Autodesk Inventor part; units mm, degrees
ref_plane "YZ Plane" through (0, 0, 0) normal (1, 0, 0) x (0, 1, 0)
ref_plane "XZ Plane" through (0, 0, 0) normal (0, 1, 0) x (-1, 0, 0)
ref_plane "XY Plane" through (0, 0, 0) normal (0, 0, 1) x (1, 0, 0)
sketch "Sketch1" plane through (0, 0, 0) normal (0, 1, 0) x (-1, 0, 0)
  line L0 (0, 0) -> (100, 0)
  line L1 (100, 0) -> (100, -50)
  line L2 (100, -50) -> (0, -50)
  line L3 (0, -50) -> (0, 0)
  line L4 (0, 0) -> (0, -16.6667)
  line L5 (0, -16.6667) -> (6, -16.6667)
  dimension "d0" = 100
  dimension "d1" = 50
  dimension "d2" = 16.6667
  dimension "d3" = 6
extrude "Extrusion1" add sketch "Sketch1" along normal blind 6
sketch "Sketch3" plane through (0, 6, 0) normal (0, 1, 0) x (1, 0, 0)
  circle A0 centre (-13, 12.5) radius 2.75
  line L0 (0, 0) -> (0, 50)
  line L1 (-100, 0) -> (0, 0)
  circle A1 centre (-13, 37.5) radius 2.75
  dimension "d21" = 5.5
  dimension "d22" = 13
  dimension "d23" = 12.5
  dimension "d26" = 25
extrude "Extrusion3" cut sketch "Sketch3" against normal through all
sketch "Sketch4" plane through (0, 6, 0) normal (0, 1, 0) x (1, 0, 0)
  circle A0 centre (-13, 12.5) radius 2.75
  line L0 (-13, 12.5) -> (-73, 12.5)
  line L1 (-73, 12.5) -> (-91, 12.5) construction
  line L2 (-73, 15.25) -> (-91, 15.25)
  line L3 (-91, 9.75) -> (-73, 9.75)
  arc A1 (-73, 9.75) -> (-73, 15.25) centre (-73, 12.5) ccw
  arc A2 (-91, 15.25) -> (-91, 9.75) centre (-91, 12.5) ccw
  point P0 (0, 0)
  point P1 (-82, 12.5)
  dimension "d33" = 60
  dimension "d34" = 18
  dimension "d35" = 5.5
extrude "Extrusion4" cut sketch "Sketch4" against normal through all contours A1 L3 A2 L2
pattern_linear "Rectangular Pattern2" count 2 spacing 25 along (0, 0, -1) of "Extrusion4"
sketch "Sketch5" plane through (0, 0, -50) normal (0, 0, -1) x (-1, 0, 0)
  line L0 (100, 0) -> (100, 6)
  line L1 (100, 0) -> (0, 0)
  line L2 (100, 6) -> (70, 6)
  line L3 (70, 6) -> (70, 0)
  line L4 (70, 0) -> (100, 0)
  line L5 (100, 0) -> (100, 6)
  dimension "d45" = 30
extrude "Extrusion5" add sketch "Sketch5" along normal blind 25
sketch "Sketch6" plane through (0, 6, 0) normal (0, 1, 0) x (1, 0, 0)
  line L0 (-82, 60.5) -> (-82, 70.5) construction
  line L1 (-79.25, 60.5) -> (-79.25, 70.5)
  line L2 (-84.75, 70.5) -> (-84.75, 60.5)
  arc A0 (-84.75, 60.5) -> (-79.25, 60.5) centre (-82, 60.5) ccw
  arc A1 (-79.25, 70.5) -> (-84.75, 70.5) centre (-82, 70.5) ccw
  line L3 (-70, 50) -> (-70, 75)
  arc A2 (-91, 40.25) -> (-91, 34.75) centre (-91, 37.5) ccw
  point P0 (0, 0)
  point P1 (-82, 65.5)
  dimension "d48" = 10
  dimension "d49" = 5.5
  dimension "d50" = 12
  dimension "d51" = 28
extrude "Extrusion6" cut sketch "Sketch6" against normal through all
fillet "Fillet2" radius 5 6 edges at (-100, 3, 0) (0, 3, 0) (-70, 3, -75) (-100, 3, -75) (0, 3, -50) (-70, 3, -50)
sketch "Sketch7" plane through (0, 6, 0) normal (0, 1, 0) x (1, 0, 0)
  circle A0 centre (-13, 12.5) radius 2.75
  line L0 (-13, 12.5) -> (-35, 12.5)
  line L1 (-35, 12.5) -> (-55, 12.5)
  circle A1 centre (-55, 12.5) radius 2.75
  circle A2 centre (-35, 12.5) radius 2.75
  line L2 (0, 5) -> (0, 45)
  line L3 (0, 0) -> (0, 45)
  circle A3 centre (-35, 37.5) radius 2.75
  circle A4 centre (-55, 37.5) radius 2.75
  dimension "d55" = 22
  dimension "d56" = 20
  dimension "d57" = 5.5
  dimension "d58" = 5.5
  dimension "d61" = 25
extrude "Extrusion7" cut sketch "Sketch7" against normal through all contours A1 | A2 L1 L0 | L0 L1 A2 | A3 | A4
sketch "Sketch9" plane through (0, 6, 0) normal (0, 1, 0) x (1, 0, 0)
  point P0 (0, 0)
properties part number "X_Carriage_Plate"
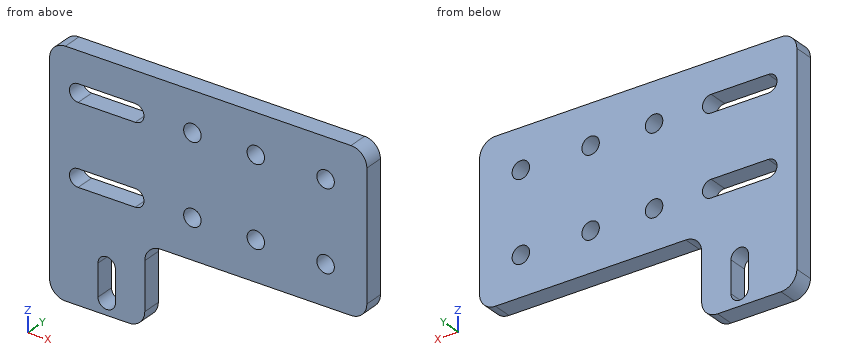
Geometry check sheet. Reference: the model listing, model coordinates, mm. Coordinates: 2 decimals unless noted, no trailing zeros. Write each loop counter-clockwise with the first axis right and the second up, starting at its lowest first coordinate (ties: lowest second). Pieces come first, ordered by that corner, then holes. Notation, with made-up numbers: M 82,73 L 88,73 A15 ccw 88,80 Z; hole C 39.5,81.25 d5. An arc over 180 degrees is marked long. Use one line per item in the form item = value. Start each with the question number.
1) Section check C-C on y = 1.1. State how many separate pieces and enclosed holes the cut face has, and give its area (3 significant figures).
2) Section check B-B on x = -82. Enter the section's corners in (y, z), and give its area (3 significant figures).
3) Section check A-A on z = -12.5. Enter the section's corners in (x, y).
4) Go/stop test with flat-tipped pins: pin 1 Ø5 at (x, z) = (-55, -37.5) entering from +Y; pin 2 Ø3 at (x, y) = (-22, 4) entering from -Z; pin 3 Ø1.8 at (y, z) = (4.5, -66) entering from +X. Record where each tip stops, or that it passes through.
5) Section check D-D on x = -25. Enter the section's corners in (y, z).
6) Thickness scan on probe 1 along Z at (x, y) = (-55, 2.1); probe 2 along X at (y, z) = (4.15, -12.5); probe 3 along Z at (x, y) = (-72, 3.7). Record the ranges inside material, lowest first. Write a range as from..to.
Responses:
q1.separate_pieces = 1
q1.enclosed_holes = 9
q1.area = 5,260 mm2
q2.outline = M 0,-75 L 6,-75 L 6,-73.25 L 0,-73.25 Z; M 0,-57.75 L 6,-57.75 L 6,-40.25 L 0,-40.25 Z; M 0,-34.75 L 6,-34.75 L 6,-15.25 L 0,-15.25 Z; M 0,-9.75 L 6,-9.75 L 6,0 L 0,0 Z
q2.area = 291 mm2
q3.outline = M -100,0 L -93.75,0 L -93.75,6 L -100,6 Z; M -70.25,0 L -57.75,0 L -57.75,6 L -70.25,6 Z; M -52.25,0 L -37.75,0 L -37.75,6 L -52.25,6 Z; M -32.25,0 L -15.75,0 L -15.75,6 L -32.25,6 Z; M -10.25,0 L 0,0 L 0,6 L -10.25,6 Z
q4.pin_1 = through
q4.pin_2 = -50
q4.pin_3 = -70
q5.outline = M 0,-50 L 6,-50 L 6,0 L 0,0 Z
q6.probe_1 = -50..-40.25, -34.75..-15.25, -9.75..0
q6.probe_2 = -100..-93.75, -70.25..-57.75, -52.25..-37.75, -32.25..-15.75, -10.25..0
q6.probe_3 = -74..-40.06, -34.94..-15.06, -9.94..0
